from build123d import *

# Parameters (mm, degrees)
SKETCH_1_W          = 10
SKETCH_1_H          = 10
SKETCH_1_W_2        = 8
SKETCH_1_H_2        = 8
EXTRUDE_1_DEPTH     = 37
SKETCH_2_R          = 1.5
CUT_EXTRUDE_1_DEPTH = 10


with BuildPart() as part:
    # 草图1 → 拉伸-薄壁1 (new body)
    with BuildSketch(Plane.XY):
        with Locations((12.317764791, -104.586504738)):
            Rectangle(SKETCH_1_W, SKETCH_1_H)
        with Locations((12.317764791, -104.586504738)):
            Rectangle(SKETCH_1_W_2, SKETCH_1_H_2, mode=Mode.SUBTRACT)
    extrude(amount=EXTRUDE_1_DEPTH)

    # 草图2 → 切除-拉伸1 (cut)
    with BuildSketch(Plane.XZ.offset(109.586504738)):
        with Locations((12.317764791, 5)):
            Circle(SKETCH_2_R)
        with Locations((12.317764791, 32)):
            Circle(SKETCH_2_R)
    extrude(amount=-CUT_EXTRUDE_1_DEPTH, mode=Mode.SUBTRACT)


solid = part.part
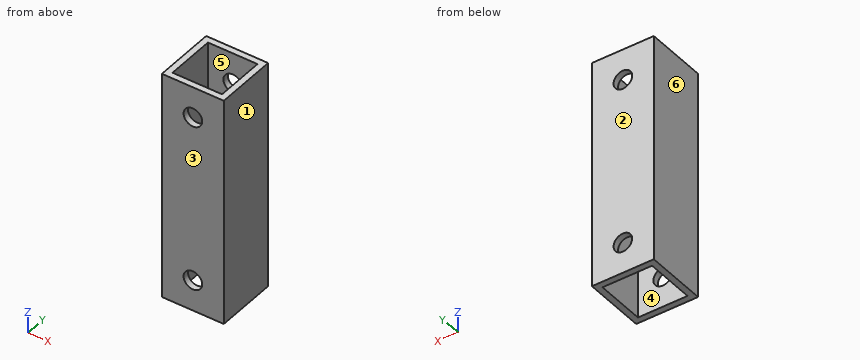
Geometry: final body of the model. Coordinates: model frame, mm. Face numbers are marked on the shaded views. A direction names the side the tool comes from. Coordinates: 2 decimals unless noted, no trailing zeros. Order: outer loops, then holes, each group sorted by start corner. A loop starts at its lowest first (then second) coordinate and runs counter-clockwise, first axis right, second up.
(1) Section query C-C (z = 3). Return the cut outline in (x, y).
(2) Section query D-D (y = -100.25). Return the cut outline in (x, z).
(3) Material intervals for probe 1 along Y at (x, z) = (14, 7); probe 2 along X at (y, z) = (-108, 6.5), sorted ascending.
(4) Access query for the marked faces 5 and 6. Directions: +Z, -Z, +X, -X, +Y, -Y. A direction counts if a zero-diameter tool reaches every point of the face in a straight line with its end or side. Return the directions, or none.
(5) Section query A-A (y = -103.75). Return the cut outline in (x, z).
(6) Draft query along Y for the marked faces 1, 2, 3 and 4. Return one class per face: pulls with the +Y half, pulls with the -Y half, needs draft (parallel to the pull), parting line crosses it, or undercut.
(7) First-contact query: pin 1 (2 mm diameter, centred on x = 13.5, y = -106, fed in from -Z); pin 2 (5 mm diameter, centred on x = 12.32, z = 32, fed in from +Y). Flat tips, straight axial feed; report the tip coordinate or a pass-through.
(8) Section query B-B (x = 8.75). Return the cut outline in (y, z), plus the area to 3 significant figures.
Solution:
1. outline: (7.32, -109.59) - (17.32, -109.59) - (17.32, -99.59) - (7.32, -99.59) - close; hole (8.32, -108.59) - (16.32, -108.59) - (16.32, -100.59) - (8.32, -100.59) - close
2. outline: (7.32, 0) - (17.32, 0) - (17.32, 37) - (7.32, 37) - close; hole circle Ø3 at (12.32, 5); hole circle Ø3 at (12.32, 32)
3. probe 1: y = -109.59 to -108.59, -100.59 to -99.59
3. probe 2: x = 7.32 to 8.32, 16.32 to 17.32
4. face 5: +Z, -Z
4. face 6: +Z, -Z, -X, +Y, -Y
5. outline: (7.32, 0) - (8.32, 0) - (8.32, 37) - (7.32, 37) - close; (16.32, 0) - (17.32, 0) - (17.32, 37) - (16.32, 37) - close
6. face 1: needs draft
6. face 2: pulls with the +Y half
6. face 3: pulls with the -Y half
6. face 4: undercut
7. pin 1: passes through
7. pin 2: stops at y = -99.59
8. outline: (-109.59, 0) - (-108.59, 0) - (-108.59, 37) - (-109.59, 37) - close; (-100.59, 0) - (-99.59, 0) - (-99.59, 37) - (-100.59, 37) - close
8. area: 74.0 mm2
